Verification items for the finished model (mm, model axes). Coordinates: 2 decimals unless noted, no trailing zeros. Loops run counter-clockwise (first coordinate to the right, second up) from the corner with the lowest first, then second, coordinate; pieces in that order, holes last. Notation, with made-up numbers: (86, 14.5) -> (115, 14.5) arc R8 ccw to (115, 29.5) -> close; hole circle Ø1 at (25, -32). An arc over 180 degrees is marked (long way). Write item = value, one per line.
```python
from build123d import *

# Parameters (mm, degrees)
F0_W     = 100.33
F0_H     = 100.33
F1_DEPTH = 7.62
F2_W     = 22.225
F2_H     = 22.225
F3_DEPTH = 2.54
F5_W     = 25.4
F5_H     = 3.81
F6_DEPTH = 2.54
F4_W     = 25.4
F4_H     = 3.81
F7_DEPTH = 2.54


with BuildPart() as f1:
    # F0 (on Top) → F1 (new body)
    with BuildSketch(Plane.XY):
        with Locations((50.165, 50.165)):
            Rectangle(F0_W, F0_H)
    extrude(amount=-F1_DEPTH)

    # F2 (on Top) → F3 (cut)
    with BuildSketch(Plane.XY):
        with Locations((13.6525, 86.6775)):
            Rectangle(F2_W, F2_H)
        with Locations((38.4175, 86.6775)):
            Rectangle(F2_W, F2_H)
        with Locations((63.1825, 86.6775)):
            Rectangle(F2_W, F2_H)
        with Locations((87.9475, 86.6775)):
            Rectangle(F2_W, F2_H)
        with Locations((13.6525, 61.9125)):
            Rectangle(F2_W, F2_H)
        with Locations((13.6525, 37.1475)):
            Rectangle(F2_W, F2_H)
        with Locations((13.6525, 12.3825)):
            Rectangle(F2_W, F2_H)
        with Locations((38.4175, 61.9125)):
            Rectangle(F2_W, F2_H)
        with Locations((63.1825, 61.9125)):
            Rectangle(F2_W, F2_H)
        with Locations((87.9475, 61.9125)):
            Rectangle(F2_W, F2_H)
        with Locations((38.4175, 37.1475)):
            Rectangle(F2_W, F2_H)
        with Locations((38.4175, 12.3825)):
            Rectangle(F2_W, F2_H)
        with Locations((63.1825, 37.1475)):
            Rectangle(F2_W, F2_H)
        with Locations((87.9475, 37.1475)):
            Rectangle(F2_W, F2_H)
        with Locations((63.1825, 12.3825)):
            Rectangle(F2_W, F2_H)
        with Locations((87.9475, 12.3825)):
            Rectangle(F2_W, F2_H)
    extrude(amount=-F3_DEPTH, mode=Mode.SUBTRACT)

    # F5 (on face) → F6 (join)
    with BuildSketch(Plane.YZ.offset(100.33)):
        with Locations((50.165, -3.81)):
            Rectangle(F5_W, F5_H)
    extrude(amount=F6_DEPTH)

    # F4 (on face) → F7 (join)
    with BuildSketch(Plane.XZ):
        with Locations((50.165, -3.81)):
            Rectangle(F4_W, F4_H)
    extrude(amount=F7_DEPTH)


solid = f1.part
```
1) Sectioned sample at A-A, the plane x = 18. Record the cut outline in (y, z) (3 decimals).
Ans:
outline = (0, -7.62) -> (100.33, -7.62) -> (100.33, 0) -> (97.79, 0) -> (97.79, -2.54) -> (75.565, -2.54) -> (75.565, 0) -> (73.025, 0) -> (73.025, -2.54) -> (50.8, -2.54) -> (50.8, 0) -> (48.26, 0) -> (48.26, -2.54) -> (26.035, -2.54) -> (26.035, 0) -> (23.495, 0) -> (23.495, -2.54) -> (1.27, -2.54) -> (1.27, 0) -> (0, 0) -> close
2) Sectioned sample at C-C, the plane y = 45.5. Record the cut outline in (x, z) (3 decimals), plus the area to 3 significant figures.
Ans:
outline = (0, -7.62) -> (100.33, -7.62) -> (100.33, -5.715) -> (102.87, -5.715) -> (102.87, -1.905) -> (100.33, -1.905) -> (100.33, 0) -> (99.06, 0) -> (99.06, -2.54) -> (76.835, -2.54) -> (76.835, 0) -> (74.295, 0) -> (74.295, -2.54) -> (52.07, -2.54) -> (52.07, 0) -> (49.53, 0) -> (49.53, -2.54) -> (27.305, -2.54) -> (27.305, 0) -> (24.765, 0) -> (24.765, -2.54) -> (2.54, -2.54) -> (2.54, 0) -> (0, 0) -> close
area = 548 mm2
3) Sectioned sample at D-D, the plane y = 35. Record the cut outline in (x, z) (3 decimals).
Ans:
outline = (0, -7.62) -> (100.33, -7.62) -> (100.33, 0) -> (99.06, 0) -> (99.06, -2.54) -> (76.835, -2.54) -> (76.835, 0) -> (74.295, 0) -> (74.295, -2.54) -> (52.07, -2.54) -> (52.07, 0) -> (49.53, 0) -> (49.53, -2.54) -> (27.305, -2.54) -> (27.305, 0) -> (24.765, 0) -> (24.765, -2.54) -> (2.54, -2.54) -> (2.54, 0) -> (0, 0) -> close
4) Depth check by flat-ended pin: pin 1 Ø3 at (x, z) = (101.5, -3) entering from -Y; pin 2 Ø4 at (y, z) = (32, -5.5) entering from +X; pin 3 Ø6.5 at (x, y) = (37.5, 84.5) entering from +Z. Enter the tip coordinate at first touch or a pass-through.
Ans:
pin_1 = 0
pin_2 = 100.33
pin_3 = -2.54
5) Material ranges on line 1 (Y direction, x = 98.5, z = -0.5) (3 decimals); line 2 (X direction, y = 3, z = -2.5) (3 decimals); line 3 (Y direction, x = 46.5, z = -2.5) (3 decimals), recorded low to high.
Ans:
line_1 = 0 to 1.27, 23.495 to 26.035, 48.26 to 50.8, 73.025 to 75.565, 97.79 to 100.33
line_2 = 0 to 2.54, 24.765 to 27.305, 49.53 to 52.07, 74.295 to 76.835, 99.06 to 100.33
line_3 = -2.54 to 1.27, 23.495 to 26.035, 48.26 to 50.8, 73.025 to 75.565, 97.79 to 100.33
6) Sectioned sample at B-B, the plane z = -4.25. Record the cut outline in (x, y) (3 decimals), plus the area to 3 significant figures.
Ans:
outline = (0, 0) -> (37.465, 0) -> (37.465, -2.54) -> (62.865, -2.54) -> (62.865, 0) -> (100.33, 0) -> (100.33, 37.465) -> (102.87, 37.465) -> (102.87, 62.865) -> (100.33, 62.865) -> (100.33, 100.33) -> (0, 100.33) -> close
area = 10,200 mm2
